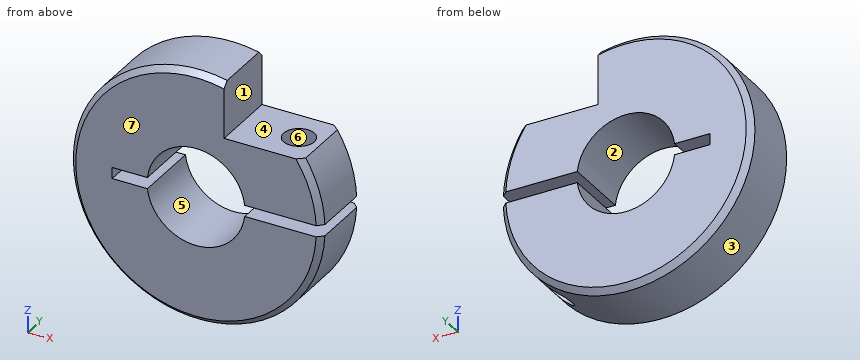
```python
from build123d import *

# Parameters (mm, degrees)
SKETCH_1_R                  = 22.5
EXTRUDE_1_DEPTH             = 6
HOLE_WIZARD_M20_1_D         = 17.5
SKETCH_2_W                  = 37.5
SKETCH_2_H                  = 2
CUT_EXTRUDE_1_DEPTH         = 35.007352146
CUT_EXTRUDE_2_DEPTH         = 35.007352146
HOLE_WIZARD_5_5_5_5_1_D     = 5.5
HOLE_WIZARD_5_5_5_5_1_DEPTH = 11
HOLE_WIZARD_M5_2_D          = 4.2
CHAMFER_1_SIZE              = 1


with BuildPart() as part:
    # 草图1 → 凸台-拉伸1 (new, symmetric)
    with BuildSketch(Plane(origin=(0, 0, 0), x_dir=(1, 0, 0), z_dir=(0, 1, 0))):
        with Locations(Location((0, 0, 0), (0, 0, 270))):
            Circle(SKETCH_1_R)
    extrude(amount=EXTRUDE_1_DEPTH, both=True)

    # M20 螺纹孔1 (through all)
    with Locations(Plane(origin=(0, 6, 0), x_dir=(1, 0, 0), z_dir=(0, 1, 0))):
        with Locations((0, 0)):
            Hole(HOLE_WIZARD_M20_1_D / 2)

    # 草图2 → 切除-拉伸1 (cut, through all)
    with BuildSketch(Plane(origin=(0, 6, 0), x_dir=(1, 0, 0), z_dir=(0, 1, 0))):
        with Locations((3.75, 0)):
            Rectangle(SKETCH_2_W, SKETCH_2_H)
    extrude(amount=-CUT_EXTRUDE_1_DEPTH, mode=Mode.SUBTRACT)

    # 草图6 → 切除-拉伸2 (cut, through all)
    with BuildSketch(Plane(origin=(0, 6, 0), x_dir=(1, 0, 0), z_dir=(0, 1, 0))):
        with BuildLine():
            Line((19.032866311, -12), (5, -12))
            Line((5, -12), (5, -21.937410968))
            ThreePointArc((5, -21.937410968), (13.003180379, -18.362115892), (19.032866311, -12))
        make_face()
    extrude(amount=-CUT_EXTRUDE_2_DEPTH, mode=Mode.SUBTRACT)

    # Ø5.5 (5.5) 直径孔1
    with Locations(Plane.XY.offset(12)):
        with Locations((15, 0)):
            Hole(HOLE_WIZARD_5_5_5_5_1_D / 2, depth=HOLE_WIZARD_5_5_5_5_1_DEPTH)

    # M5 螺纹孔2 (through all)
    with Locations(Plane(origin=(-28, -6, -1), x_dir=(1, 0, 0), z_dir=(0, 0, 1))):
        with Locations((43, 6)):
            Hole(HOLE_WIZARD_M5_2_D / 2)

    # 倒角1
    chamfer_1_edges = [part.edges().sort_by_distance(p)[0] for p in [
        (-17.896595276, -6, -13.636783988),
        (-17.896595276, 6, -13.636783988),
        (21.471682868, -6, 6.724346424),
        (21.471682868, 6, 6.724346424),
    ]]
    chamfer(chamfer_1_edges, length=CHAMFER_1_SIZE)


solid = part.part
```
CAD build for the part. Positions are in the model's coordinates, mm. Face numbers are marked on the shaded views. A direction names the side the tool comes from. Coordinates: 2 decimals unless noted, no trailing zeros. Order: outer loops, then holes, each group sorted by start corner. A loop starts at its lowest first (then second) coordinate and runs counter-clockwise, first axis right, second up.
(1) Saw through at A-A, the plane x = 0. Write the cut outline in (y, z).
Solution:
outline: (-6, -21.5) - (-5, -22.5) - (5, -22.5) - (6, -21.5) - (6, -8.75) - (-6, -8.75) - close; (-6, 8.75) - (6, 8.75) - (6, 21.5) - (5, 22.5) - (-5, 22.5) - (-6, 21.5) - close
(2) Saw through at B-B, the plane y = -1.25. Write the cut outline in (x, z), and give its area (3 significant figures).
Solution:
outline: (-15, -1) - (-15, 1) - (-8.69, 1) arc R8.75 cw to (8.69, 1) - (12.55, 1) - (12.55, 12) - (5, 12) - (5, 21.94) arc R22.5 ccw (long way) to (13.31, -18.14) - (13.31, -1) - (8.69, -1) arc R8.75 cw to (-8.69, -1) - close; (16.69, -15.09) arc R22.5 ccw to (22.48, -1) - (16.69, -1) - close; (17.45, 1) - (22.48, 1) arc R22.5 ccw to (19.03, 12) - (17.45, 12) - close
area: 1,110 mm2
(3) Saw through at D-D, the plane x = 15. Count the separate pieces of the cut face and the enclosed holes in it, and give its area (3 significant figures).
Solution:
separate pieces: 4
enclosed holes: 0
area: 193 mm2
(4) Which spindle directions (+Z, -Z, +X, -X, +Y, -Y) get a long thin tool onto all of the face, cutting with end or side? Do the marked faces 4, 5, 6 and 7. Say none if no direction does.
Solution:
face 4: +Z, +X, +Y, -Y
face 5: +Y, -Y
face 6: +Z
face 7: +Z, -Z, +X, -X, -Y
(5) Saw through at C-C, the plane z = 0. Write the cut outline in (x, y).
Solution:
outline: (-22.5, -5) - (-21.5, -6) - (-15, -6) - (-15, 6) - (-21.5, 6) - (-22.5, 5) - close
(6) Drill centre lines: L1, parallel to Y at x = 15, z = -8.5; L2, parallel to Y at x = 15, z = 6; L3, parallel to Z at x = -9, y = -3. Where is each one in solid material? Low to high.
Solution:
L1: y = -6 to -2.1, 2.1 to 6
L2: y = -6 to -2.75, 2.75 to 6
L3: z = -20.62 to -1, 1 to 20.62
(7) Mould opens along X. For the marked faces 1, 2 and 3 say: released by +X, released by -X, zero draft, split by the parting line, or undercut.
Solution:
face 1: released by +X
face 2: undercut
face 3: split by the parting line
(8) Pin check, flat tips, straight feed: pin 1 Ø6 at (x, y) = (14, -1) entering from +Z; pin 2 Ø1.5 at (y, z) = (-4.5, 2.5) entering from -X; pin 3 Ø1 at (y, z) = (0, 6.5) entering from +X. Stop position of each tip, or through.
Solution:
pin 1: stops at z = 12
pin 2: stops at x = -22.43
pin 3: stops at x = 21.69
